Read the model definition and answer for the solid it produces. Units are mm, in the model's axes. A direction names the side the tool comes from. Coordinates: 2 decimals unless noted, no trailing zeros. Loops run counter-clockwise (first coordinate to the right, second up) from the corner with the lowest first, then second, coordinate; pieces in that order, holes last.
from build123d import *

# Parameters (mm, degrees)
SM_BASE_FLANGE_1_DEPTH   = 80
CUT_EXTRUDE_3_DEPTH      = 109.411254028
CUT_EXTRUDE_3_DEPTH_BACK = 109.411254028
SKETCH_6_R               = 48
SKETCH_6_R_2             = 2
FILLET_1_R               = 5
SKETCH_9_R               = 2
CUT_EXTRUDE_4_DEPTH      = 93.287593966


# Sheet-metal steps are written as plain solids
with BuildPart() as part:
    # Sketch 1 → Базовая кромка1 (new body)
    with BuildSketch(Plane.XY):
        with BuildLine():
            Line((-30, 27), (-30, 1))
            ThreePointArc((-30, 1), (-29.707106781, 0.292893219), (-29, 0))
            Line((-29, 0), (29, 0))
            ThreePointArc((29, 0), (29.707106781, 0.292893219), (30, 1))
            Line((30, 1), (30, 27))
            Line((30, 27), (34, 27))
            Line((34, 27), (34, 1))
            ThreePointArc((34, 1), (32.535533906, -2.535533906), (29, -4))
            Line((29, -4), (-29, -4))
            ThreePointArc((-29, -4), (-32.535533906, -2.535533906), (-34, 1))
            Line((-34, 1), (-34, 27))
            Line((-34, 27), (-30, 27))
        make_face()
    extrude(amount=SM_BASE_FLANGE_1_DEPTH)

    # Эскиз6 → Вырез-Вытянуть3 (cut, two sides: drawn at the far end of the back side and taken through both)
    with BuildSketch(Plane.ZY.offset(34).offset(-CUT_EXTRUDE_3_DEPTH_BACK)):
        with Locations((40, 65)):
            Circle(SKETCH_6_R)
        with Locations((40, 12)):
            Circle(SKETCH_6_R_2)
        with Locations((8.847381628, 22.122099298)):
            Circle(SKETCH_6_R_2)
        with Locations((71.152618372, 22.122099298)):
            Circle(SKETCH_6_R_2)
    extrude(amount=CUT_EXTRUDE_3_DEPTH + CUT_EXTRUDE_3_DEPTH_BACK, mode=Mode.SUBTRACT)

    # Скругление1
    fillet_1_edges = [part.edges().sort_by_distance(p)[0] for p in [
        (32, 27, 10.674243403),
        (32, 27, 69.325756597),
        (-32, 27, 10.674243403),
        (-32, 27, 69.325756597),
    ]]
    fillet(fillet_1_edges, radius=FILLET_1_R)

    # Эскиз9 → Вырез-Вытянуть4 (cut, through all)
    with BuildSketch(Plane.XZ.offset(4)):
        with Locations((-21.75, 40)):
            Circle(SKETCH_9_R)
        with Locations((-10.875, 58.836052532)):
            Circle(SKETCH_9_R)
        with Locations((10.875, 58.836052532)):
            Circle(SKETCH_9_R)
        with Locations((21.75, 40)):
            Circle(SKETCH_9_R)
        with Locations((10.875, 21.163947468)):
            Circle(SKETCH_9_R)
        with Locations((-10.875, 21.163947468)):
            Circle(SKETCH_9_R)
    extrude(amount=-CUT_EXTRUDE_4_DEPTH, mode=Mode.SUBTRACT)


solid = part.part
Item 1: A cutting plane is placed at B-B on x = -21.75. Determine the outline of the cut face in (y, z).
Numbers:
outline: (-4, 0) - (0, 0) - (0, 38) - (-4, 38) - close; (-4, 42) - (0, 42) - (0, 80) - (-4, 80) - close
Item 2: Find the intervals of material crossed by line 1 along X through (y, z) = (2, 67); line 2 along Z through (x, y) = (32.35, 12); line 3 along Y through (x, z) = (-15, 26), in increasing order.
Numbers:
line 1: x = -34 to -30, 30 to 34
line 2: z = 0 to 38, 42 to 80
line 3: y = -4 to 0
Item 3: A cutting plane is placed at D-D on z = 74.5. Determine the outline of the cut face in (x, y).
Numbers:
outline: (-34, 1) arc R5 ccw to (-29, -4) - (29, -4) arc R5 ccw to (34, 1) - (34, 27) - (30, 27) - (30, 1) arc R1 cw to (29, 0) - (-29, 0) arc R1 cw to (-30, 1) - (-30, 27) - (-34, 27) - close
Item 4: Given pin 1 (17.5 mm diameter, centred on x = -13, z = 48, fed in from +Y), flat-ended and moving along its own axis, determine where the tip first touches the part or whether it passes through.
Numbers:
pin 1: stops at y = 0
Item 5: Which of the six approach directions +Z, -Z, +X, -X, +Y, -Y give full straight-line access (tool end or side, diameter ignored) to faces 1 (the face through (-30, 14, 39)), 2 (the face through (-32, 27, 4)), 3 (the face through (32.028, 26.765, 69.469))?
Numbers:
face 1: +Z, -Z, +Y
face 2: +Z, -Z, +X, -X, +Y
face 3: +X, -X, +Y
Item 6: Determine the mould class of faces 4 (the face through (0, -1, 80)), 5 (the face through (21.316, -2.028, 38.048)), 6 (the face through (32, 27, 75)) for opening direction Z: released by +Z, released by -Z, zero draft, split by the parting line, or undercut.
Numbers:
face 4: released by +Z
face 5: undercut
face 6: zero draft
Item 7: A cutting plane is placed at C-C on z = 40. Determine the outline of the cut face in (x, y), then the cut area to 3 significant figures.
Numbers:
outline: (-34, 1) arc R5 ccw to (-29, -4) - (-23.75, -4) - (-23.75, 0) - (-29, 0) arc R1 cw to (-30, 1) - (-30, 10) - (-34, 10) - close; (-34, 14) - (-30, 14) - (-30, 17) - (-34, 17) - close; (-19.75, -4) - (19.75, -4) - (19.75, 0) - (-19.75, 0) - close; (23.75, -4) - (29, -4) arc R5 ccw to (34, 1) - (34, 10) - (30, 10) - (30, 1) arc R1 cw to (29, 0) - (23.75, 0) - close; (30, 14) - (34, 14) - (34, 17) - (30, 17) - close
area: 334 mm2
Item 8: A cutting plane is placed at A-A on y = 2.5. Determine the outline of the cut face in (x, z).
Numbers:
outline: (-34, 0) - (-30, 0) - (-30, 80) - (-34, 80) - close; (30, 0) - (34, 0) - (34, 80) - (30, 80) - close
